```python
from build123d import *

# Parameters (mm, degrees)
ESQUISSE1_R             = 16
BOSS_EXTRU_1_DEPTH      = 9.03
ESQUISSE2_R             = 15
ENL_V_MAT_EXTRU_1_DEPTH = 8
ESQUISSE3_R             = 7.5
BOSS_EXTRU_2_DEPTH      = 5
ESQUISSE4_R             = 7
BOSS_EXTRU_3_DEPTH      = 1
ESQUISSE5_R             = 6.5
BOSS_EXTRU_4_DEPTH      = 2.7
BOSS_EXTRU_5_DEPTH      = 3
BOSS_EXTRU_5_DEPTH_BACK = 0.5
ESQUISSE6_R             = 1
BOSS_EXTRU_9_DEPTH      = 12


with BuildPart() as part:
    # Esquisse1 → Boss.-Extru.1 (new body)
    with BuildSketch(Plane.XY):
        Circle(ESQUISSE1_R)
    extrude(amount=BOSS_EXTRU_1_DEPTH)

    # Esquisse2 → Enlèv. mat.-Extru.1 (cut)
    with BuildSketch(Plane.XY.offset(9.03)):
        Circle(ESQUISSE2_R)
    extrude(amount=-ENL_V_MAT_EXTRU_1_DEPTH, mode=Mode.SUBTRACT)

    # Esquisse3 → Boss.-Extru.2 (add)
    with BuildSketch(Plane(origin=(0, 0, 0), x_dir=(-1, 0, 0), z_dir=(0, 0, -1))):
        with Locations(Location((0, 0, 0), (0, 0, 180))):
            Circle(ESQUISSE3_R)
    extrude(amount=BOSS_EXTRU_2_DEPTH)

    # Esquisse4 → Boss.-Extru.3 (add)
    with BuildSketch(Plane(origin=(0, 0, -5), x_dir=(-1, 0, 0), z_dir=(0, 0, -1))):
        Circle(ESQUISSE4_R)
    extrude(amount=BOSS_EXTRU_3_DEPTH)

    # Esquisse5 → Boss.-Extru.4 (add)
    with BuildSketch(Plane(origin=(0, 0, -6), x_dir=(-1, 0, 0), z_dir=(0, 0, -1))):
        with Locations(Location((0, 0, 0), (0, 0, 180))):
            Circle(ESQUISSE5_R)
    extrude(amount=BOSS_EXTRU_4_DEPTH)

    # Esquisse6 → Boss.-Extru.5 (add, two sides: drawn at the far end of the back side and taken through both)
    with BuildSketch(Plane(origin=(0, 16, 0), x_dir=(-1, 0, 0), z_dir=(0, 1, 0)).offset(-BOSS_EXTRU_5_DEPTH_BACK)):
        with Locations(Location((1.1, 4.857681609, 0), (0, 0, 90))):
            Circle(ESQUISSE6_R)
        with Locations(Location((-1.1, 4.857681609, 0), (0, 0, 90))):
            Circle(ESQUISSE6_R)
    extrude(amount=BOSS_EXTRU_5_DEPTH + BOSS_EXTRU_5_DEPTH_BACK)

    # Esquisse7 → Boss.-Extru.9 (add)
    with BuildSketch(Plane(origin=(0, 16, 0), x_dir=(-1, 0, 0), z_dir=(0, 1, 0))):
        with BuildLine():
            ThreePointArc((2.218175405, -7.992904998), (3.268175405, -7.763776214), (2.218175405, -7.534647429))
            ThreePointArc((2.218175405, -7.534647429), (1.718175405, -7.213776214), (1.218175405, -7.534647429))
            ThreePointArc((1.218175405, -7.534647429), (0.718175405, -7.213776214), (0.218175405, -7.534647429))
            ThreePointArc((0.218175405, -7.534647429), (-0.281824595, -7.213776214), (-0.781824595, -7.534647429))
            ThreePointArc((-0.781824595, -7.534647429), (-1.281824595, -7.213776214), (-1.781824595, -7.534647429))
            ThreePointArc((-1.781824595, -7.534647429), (-2.831824595, -7.763776214), (-1.781824595, -7.992904998))
            ThreePointArc((-1.781824595, -7.992904998), (-1.281824595, -8.313776214), (-0.781824595, -7.992904998))
            ThreePointArc((-0.781824595, -7.992904998), (-0.281824595, -8.313776214), (0.218175405, -7.992904998))
            ThreePointArc((0.218175405, -7.992904998), (0.718175405, -8.313776214), (1.218175405, -7.992904998))
            ThreePointArc((1.218175405, -7.992904998), (1.718175405, -8.313776214), (2.218175405, -7.992904998))
        make_face()
    extrude(amount=-BOSS_EXTRU_9_DEPTH)


solid = part.part
```
Build history of the part. All positions in model axes, mm. A direction names the side the tool comes from. Round coordinates to 2 decimals unless told otherwise and drop trailing zeros. Order: outer loops, then holes, each group sorted by start corner. A loop starts at its lowest first (then second) coordinate and runs counter-clockwise, first axis right, second up. Notation, with made-up numbers: (55.25, 33) -> (75.25, 33) arc R6 cw to (75.25, 41) -> close; hole circle Ø1 at (60, -6). An arc over 180 degrees is marked (long way). Answer in a Markdown table with one row per item.
1) Mould opens along Y. For faces 3 (the cylindrical face through (-14.985, 0.66, 5.086)), 4 (the flat face through (-1, 19, 5)), 5 (the cylindrical face through (-6.466, -2.681, -5.493)), 6 (the flat face through (-2, 7, -5)) say: released by +Y, released by -Y, zero draft, split by the parting line, or undercut.
Values:
| item | result |
|---|---|
| face 3 | undercut |
| face 4 | released by +Y |
| face 5 | split by the parting line |
| face 6 | zero draft |
2) Pin check, flat tips, straight feed: P1, Ø5, axis at x = 8.5, y = 14, coming from the -Z side; P2, Ø4, axis at x = 7.5, y = 0.5, coming from the +Z side; P3, Ø3, axis at y = 13.5, z = -4, coming from the +X side; P4, Ø4, axis at x = 4, z = -1.5, coming from the +Y side. Stop position of each tip, or through.
Values:
| item | result |
|---|---|
| P1 | z = 0 |
| P2 | z = 1.03 |
| P3 | through |
| P4 | y = 15.77 |
3) Band-saw the part on A-A on y = 12.5. Give the cut face in (x, z), and give its area (3 significant figures).
Values:
| item | result |
|---|---|
| outline | (-9.99, 0) -> (9.99, 0) -> (9.99, 9.03) -> (8.29, 9.03) -> (8.29, 1.03) -> (-8.29, 1.03) -> (-8.29, 9.03) -> (-9.99, 9.03) -> close; (-2.22, -7.99) arc R0.55 ccw to (-1.22, -7.99) arc R0.55 ccw to (-0.22, -7.99) arc R0.55 ccw to (0.78, -7.99) arc R0.55 ccw to (1.78, -7.99) arc R0.55 ccw (long way) to (1.78, -7.53) arc R0.55 ccw to (0.78, -7.53) arc R0.55 ccw to (-0.22, -7.53) arc R0.55 ccw to (-1.22, -7.53) arc R0.55 ccw to (-2.22, -7.53) arc R0.55 ccw (long way) to start |
| area | 53.3 mm2 |
4) Band-saw the part on D-D on y = 0. Give the cut face in (x, z), and give its area (3 significant figures).
Values:
| item | result |
|---|---|
| outline | (-16, 0) -> (-7.5, 0) -> (-7.5, -5) -> (-7, -5) -> (-7, -6) -> (-6.5, -6) -> (-6.5, -8.7) -> (6.5, -8.7) -> (6.5, -6) -> (7, -6) -> (7, -5) -> (7.5, -5) -> (7.5, 0) -> (16, 0) -> (16, 9.03) -> (15, 9.03) -> (15, 1.03) -> (-15, 1.03) -> (-15, 9.03) -> (-16, 9.03) -> close |
| area | 173 mm2 |
5) Which spindle directions (+Z, -Z, +X, -X, +Y, -Y) get a long thin tool onto all of the face, cutting with end or side? Do faces 1 (the flat face through (0, 0, -8.7)), 2 (the flat face through (0, 16, -8)). Say none if no direction does.
Values:
| item | result |
|---|---|
| face 1 | -Z, +X, -X, +Y, -Y |
| face 2 | -Z, +X, -X, +Y |
6) Wall check: L1, parallel to Y at x = 0, z = 2.75; L2, parallel to Z at x = 7.5, y = -8; L3, parallel to Z at x = -4, y = -2. Give the ranges that are in metal, low to high.
Values:
| item | result |
|---|---|
| L1 | -16 to -15, 15 to 16 |
| L2 | 0 to 1.03 |
| L3 | -8.7 to 1.03 |
7) Band-saw the part on C-C on x = 5.5. Give the cut face in (y, z), and give its area (3 significant figures).
Values:
| item | result |
|---|---|
| outline | (-15.02, 0) -> (-5.1, 0) -> (-5.1, -5) -> (-4.33, -5) -> (-4.33, -6) -> (-3.46, -6) -> (-3.46, -8.7) -> (3.46, -8.7) -> (3.46, -6) -> (4.33, -6) -> (4.33, -5) -> (5.1, -5) -> (5.1, 0) -> (15.02, 0) -> (15.02, 9.03) -> (13.96, 9.03) -> (13.96, 1.03) -> (-13.96, 1.03) -> (-13.96, 9.03) -> (-15.02, 9.03) -> close |
| area | 126 mm2 |
8) Band-saw the part on B-B on z = 5. Give the cut face in (x, y), and give its area (3 significant figures).
Values:
| item | result |
|---|---|
| outline | (-2.09, 15.86) arc R16 ccw (long way) to (2.09, 15.86) -> (2.09, 19) -> (0.11, 19) -> (0.11, 16) arc R16 ccw to (-0.11, 16) -> (-0.11, 19) -> (-2.09, 19) -> close; hole circle Ø30 at (0, 0) |
| area | 109 mm2 |
